The listing builds one solid part. Answer for the finished solid, in the listing's coordinates (mm). Face numbers are marked on the shaded views. Give positions to 0.01 mm unless a question says otherwise; leave off trailing zeros. Write each loop counter-clockwise with the first axis right and the second up, starting at its lowest first coordinate (ties: lowest second). Pieces come first, ordered by that corner, then holes. Notation, with made-up numbers: (5.5, 18) - (22.5, 18) arc R11 cw to (22.5, 23) - close; hole circle Ø11 at (45, -12.5). An arc over 180 degrees is marked (long way). Return JSON: item names as keys, results as strings.
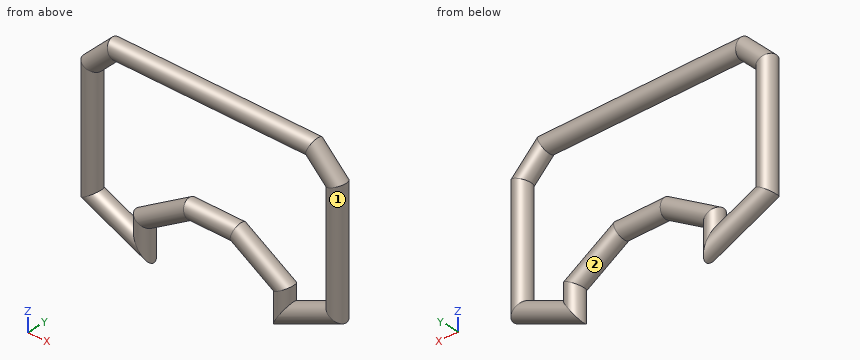
from build123d import *

# Parameters (mm, degrees)
SKETCH2_R = 19.05


with BuildPart() as part:
    # Sweep1: sweep along a path in Sketch1
    with BuildLine(Plane(origin=(0, 0, 0), x_dir=(1, 0, 0), z_dir=(0, 1, 0))) as sweep1_path:
        Line((-266.7, -373.873558028), (-266.7, -119.873558028))
        Line((-266.7, -119.873558028), (-152.4, -69.073558028))
        Line((-152.4, -69.073558028), (-152.4, -119.873558028))
        Line((-152.4, -119.873558028), (-50.8, -183.373558028))
        Line((-50.8, -183.373558028), (50.8, -183.373558028))
        Line((50.8, -183.373558028), (152.4, -119.873558028))
        Line((152.4, -119.873558028), (152.4, -69.073558028))
        Line((152.4, -69.073558028), (266.7, -119.873558028))
        Line((266.7, -119.873558028), (266.7, -373.873558028))
        Line((266.7, -373.873558028), (215.9, -424.673558028))
        Line((215.9, -424.673558028), (-215.9, -424.673558028))
        Line((-215.9, -424.673558028), (-266.7, -373.873558028))
    # Sketch2 → Sweep1 (sweep)
    with BuildSketch(Plane(origin=(0, 0, 0), x_dir=(0, 0, -1), z_dir=(1, 0, 0))):
        with Locations((-424.673558028, 0)):
            Circle(SKETCH2_R)
    sweep(path=sweep1_path.line, transition=Transition.RIGHT)


solid = part.part
Item 1: Consider L1, parallel to X at y = -3, z = 133.5; L2, parallel to Y at x = -192.5, z = 89; L3, parallel to X at y = -5, z = 152. Determine where each line is inside the solid, lowest interval first.
Answer below:
{"L1": "x = -285.51 to -247.89, -166.09 to -95.1, 95.1 to 166.09, 247.89 to 285.51", "L2": "y = -18.95 to 18.95", "L3": "x = -285.08 to -248.32, -135.68 to -66.31, 66.31 to 135.68, 248.32 to 285.08"}
Item 2: Flat-ended cylindrical pins translate along their axes: P1, Ø1, axis at y = -13.5, z = 400, coming from the +X side; P2, Ø8, axis at x = -138, y = 6.5, coming from the -Z side; P3, Ø1.5, axis at x = -85, y = 11.5, coming from the +Z side. Find the tip coordinate at first contact, or state that the pin passes through.
Answer below:
{"P1": "stops at x = 260.43", "P2": "stops at z = 40.88", "P3": "stops at z = 440.4"}
Item 3: The mould has two halves that part along X. Classify the marked faces 1 and 2: +X half, -X half, draft (parallel to the pull), parting line (faces both ways), or undercut.
Answer below:
{"face 1": "undercut", "face 2": "undercut"}
Item 4: A cutting plane is placed at A-A on y = 11.5. Determine the outline of the cut face in (x, z), then the cut area to 3 significant figures.
Answer below:
{"outline": "(-281.89, 110) - (-137.21, 45.7) - (-137.21, 111.46) - (-46.44, 168.19) - (46.44, 168.19) - (137.21, 111.46) - (137.21, 45.7) - (281.89, 110) - (281.89, 380.16) - (222.19, 439.86) - (-222.19, 439.86) - (-281.89, 380.16) - close; hole (-251.51, 129.74) - (-167.59, 92.44) - (-167.59, 128.29) - (-55.16, 198.56) - (55.16, 198.56) - (167.59, 128.29) - (167.59, 92.44) - (251.51, 129.74) - (251.51, 367.58) - (209.61, 409.49) - (-209.61, 409.49) - (-251.51, 367.58) - close", "area": "54,000 mm²"}
